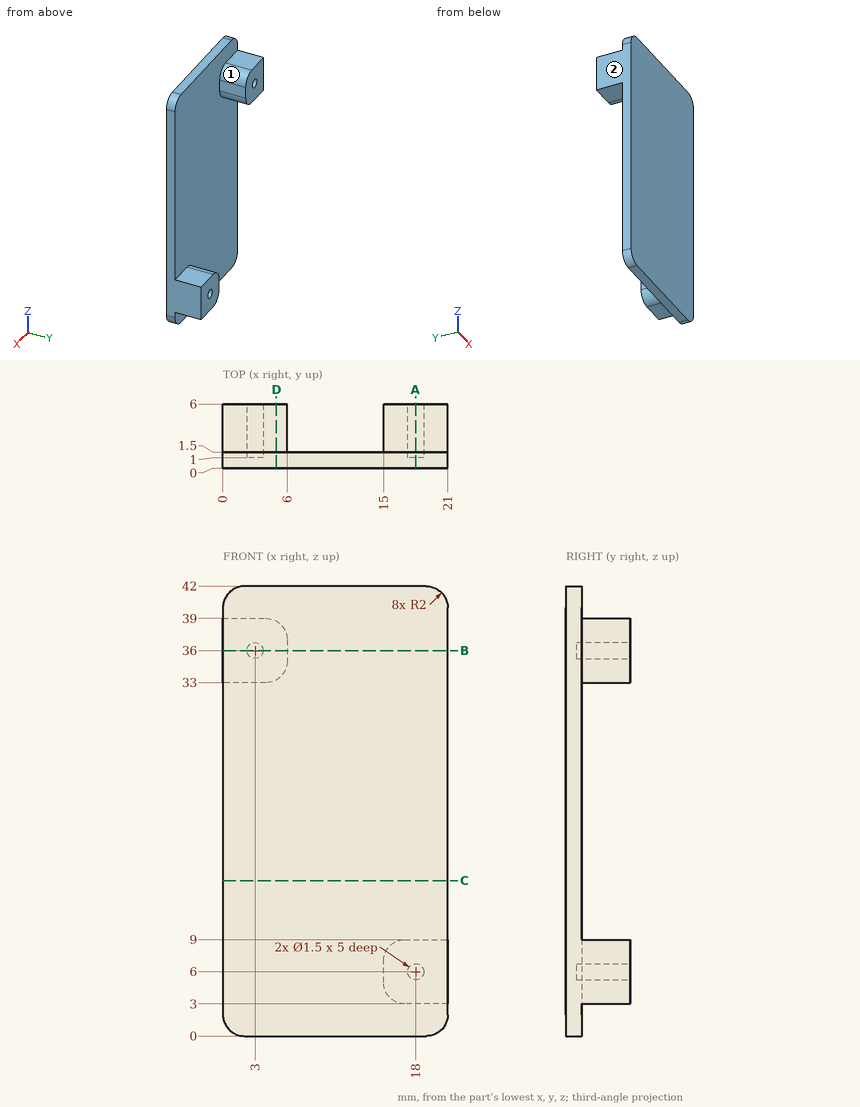
Answer from the drawing. Dimensions are ordinates in mm from the lowest x, y and z of the part. A direction names the side the tool comes from. Give positions to 0.01 mm unless a question says otherwise; leave off trailing zeros. Order: outer loops, then holes, each group sorted by start corner. A loop starts at its lowest first (then second) coordinate and runs counter-clockwise, first axis right, second up. Notation, with made-up numbers: (20, 49.5) - (27, 49.5) arc R32 cw to (27, 77.5) - close; hole circle Ø4 at (89, -28). An arc over 180 degrees is marked (long way). One line per item, written item: value. Start each with the question number.
1) A cutting plane is placed at A-A on x = 18. Give the vertices of the cut face in (y, z), then the cut area to 3 significant figures.
2) A tool of negligible diameter and unlimited length cuts with its end or side. For the marked faces 1 and 2, from which of +Z, -Z, +X, -X, +Y, -Y can it reach the whole face along a straight path? Write none if from no direction.
3) Given pin 1 Ø3 at (x, y) = (10.5, 4) entering from -Z; pin 2 Ø1.2 at (x, y) = (2, 5) entering from -Z; pin 3 Ø1 at (x, y) = (16.5, 3.5) entering from -Z; pin 4 Ø1.5 at (x, y) = (14.5, 2.5) entering from +Z, each flat-ended and moving along its own axis, determine where each tip first touches the part or whether it passes through.
4) Find the intervals of material crossed by L1, parallel to Z at x = 18, y = 5; L2, parallel to Z at x = 3, y = 2.95; L3, parallel to X at y = 3.45, z = 36, in increasing order.
5) A cutting plane is placed at C-C on z = 14.5. Give the vertices of the cut face in (x, y), then the cut area to 3 significant figures.
6) A cutting plane is placed at B-B on z = 36. Give the vertices of the cut face in (x, y).
7) A cutting plane is placed at D-D on x = 5. Give the vertices of the cut face in (y, z), then the cut area to 3 significant figures.
Answer sheet:
1. outline: (0, 0) - (1.5, 0) - (1.5, 3) - (6, 3) - (6, 5.25) - (1, 5.25) - (1, 6.75) - (6, 6.75) - (6, 9) - (1.5, 9) - (1.5, 42) - (0, 42) - close
1. area: 82.5 mm2
2. face 1: +Z, +X, +Y
2. face 2: +Z, -Z, -X, +Y, -Y
3. pin 1: passes through
3. pin 2: stops at z = 33
3. pin 3: stops at z = 3
3. pin 4: stops at z = 7.97
4. L1: z = 3 to 5.25, 6.75 to 9
4. L2: z = 33 to 35.25, 36.75 to 39
4. L3: x = 0 to 2.25, 3.75 to 6
5. outline: (0, 0) - (21, 0) - (21, 1.5) - (0, 1.5) - close
5. area: 31.5 mm2
6. outline: (0, 0) - (21, 0) - (21, 1.5) - (6, 1.5) - (6, 6) - (3.75, 6) - (3.75, 1) - (2.25, 1) - (2.25, 6) - (0, 6) - close
7. outline: (0, 0) - (1.5, 0) - (1.5, 33.27) - (6, 33.27) - (6, 38.73) - (1.5, 38.73) - (1.5, 42) - (0, 42) - close
7. area: 87.6 mm2
